Input: part model. Units: mm. Frame: model coordinates. A direction names the side the tool comes from. Round coordinates to 2 decimals unless told otherwise and drop trailing zeros. Loops run counter-clockwise (first coordinate to the right, second up) from the corner with the lowest first, then second, coordinate; pieces in that order, holes last. Notation, with made-up numbers: (-26, -22) -> (-9, -22) arc R10 ccw to (-9, -5) -> close; hole circle Ø1 at (-16.75, -0.75). An arc over 180 degrees is marked (long way). Answer as a JSON object with one key per item and string values.
```python
from build123d import *

# Parameters (mm, degrees)
SKETCH_1_R          = 2.1
SKETCH_1_R_2        = 5.02
SKETCH_1_R_3        = 2
SKETCH_1_R_4        = 9.52
EXTRUDE_1_DEPTH     = 4
SKETCH_3_W          = 46.2
SKETCH_3_H          = 3.817212264
EXTRUDE_2_DEPTH     = 4
SKETCH_2_R          = 2
SKETCH_2_R_2        = 1.5
SKETCH_2_W          = 32.809844138
SKETCH_2_H          = 42
SKETCH_2_W_2        = 8.2
SKETCH_2_H_2        = 4.2
CUT_EXTRUDE_1_DEPTH = 4
FILLET_1_R          = 2


with BuildPart() as part:
    # 草图1 → 凸台-拉伸1 (new body)
    with BuildSketch(Plane.XY):
        with BuildLine():
            ThreePointArc((-1.457142857, 39.854285714), (-41.457142857, -0.145714286), (-1.457142857, -40.145714286))
            Line((-1.457142857, -40.145714286), (328.542857143, -40.145714286))
            ThreePointArc((328.542857143, -40.145714286), (368.542857143, -0.145714286), (328.542857143, 39.854285714))
            Line((328.542857143, 39.854285714), (-1.457142857, 39.854285714))
        make_face()
        with Locations((-1.457142857, -23.895714286)):
            Circle(SKETCH_1_R, mode=Mode.SUBTRACT)
        with Locations((-20.942714442, -11.395714286)):
            Circle(SKETCH_1_R, mode=Mode.SUBTRACT)
        with Locations((18.028428728, -11.395714286)):
            Circle(SKETCH_1_R, mode=Mode.SUBTRACT)
        with Locations((-1.457142857, -0.145714286)):
            Circle(SKETCH_1_R_2, mode=Mode.SUBTRACT)
        with Locations((238.542857143, -16.645714286)):
            Circle(SKETCH_1_R_3, mode=Mode.SUBTRACT)
        with Locations((288.542857143, -0.145714286)):
            Circle(SKETCH_1_R_3, mode=Mode.SUBTRACT)
        with Locations((328.542857143, -0.145714286)):
            Circle(SKETCH_1_R_4, mode=Mode.SUBTRACT)
        with Locations((-22.025246197, 11.729285714)):
            Circle(SKETCH_1_R, mode=Mode.SUBTRACT)
        with Locations((19.110960483, 11.729285714)):
            Circle(SKETCH_1_R, mode=Mode.SUBTRACT)
        with Locations((-1.457142857, 22.354285714)):
            Circle(SKETCH_1_R, mode=Mode.SUBTRACT)
        with Locations((238.542857143, 16.354285714)):
            Circle(SKETCH_1_R_3, mode=Mode.SUBTRACT)
    extrude(amount=EXTRUDE_1_DEPTH)

    # 草图3 → 凸台-拉伸2 (add)
    with BuildSketch(Plane.XY.offset(4)):
        with Locations((18.542857143, -41.36131722)):
            Rectangle(SKETCH_3_W, SKETCH_3_H)
    extrude(amount=-EXTRUDE_2_DEPTH)

    # 草图2 → 切除-拉伸1 (cut)
    with BuildSketch(Plane.XY.offset(4)):
        with Locations((18.542857143, 33.854285714)):
            Circle(SKETCH_2_R)
        with Locations((108.542857143, 33.854285714)):
            Circle(SKETCH_2_R)
        with Locations((198.542857143, 33.854285714)):
            Circle(SKETCH_2_R)
        with Locations((288.542857143, 33.854285714)):
            Circle(SKETCH_2_R)
        with Locations((108.542857143, -34.145714286)):
            Circle(SKETCH_2_R)
        with Locations((198.542857143, -34.145714286)):
            Circle(SKETCH_2_R)
        with Locations((288.542857143, -34.145714286)):
            Circle(SKETCH_2_R)
        with Locations((18.542857143, -40.329923352)):
            Circle(SKETCH_2_R_2)
        Polygon((31.542857143, -21.145714286), (104.183898028, -21.145714286), (159.772133322, 20.854285714), (31.542857143, 20.854285714), align=None)
        Polygon((148.123425102, -21.145714286), (203.711660396, 20.854285714), (233.542857143, 20.854285714), (233.542857143, -21.145714286), align=None)
        with Locations((259.947779212, -0.145714286)):
            Rectangle(SKETCH_2_W, SKETCH_2_H)
        with Locations((33.542857143, -40.329923352)):
            Rectangle(SKETCH_2_W_2, SKETCH_2_H_2)
        with Locations((3.542857143, -40.329923352)):
            Rectangle(SKETCH_2_W_2, SKETCH_2_H_2)
    extrude(amount=-CUT_EXTRUDE_1_DEPTH, mode=Mode.SUBTRACT)

    # 圆角1
    fillet_1_edges = [part.edges().sort_by_distance(p)[0] for p in [
        (243.542857143, 20.854285714, 2),
        (276.352701281, 20.854285714, 2),
        (276.352701281, -21.145714286, 2),
        (243.542857143, -21.145714286, 2),
        (31.542857143, -21.145714286, 2),
        (31.542857143, 20.854285714, 2),
        (159.772133322, 20.854285714, 2),
        (104.183898028, -21.145714286, 2),
        (203.711660396, 20.854285714, 2),
        (233.542857143, 20.854285714, 2),
        (233.542857143, -21.145714286, 2),
        (148.123425102, -21.145714286, 2),
    ]]
    fillet(fillet_1_edges, radius=FILLET_1_R)


solid = part.part
```
1) Draft query along X for faces 1 (the face through (-41.385, 2.262, 1.972)), 2 (the face through (3.33, 1.36, 1.97)), 3 (the face through (368.533, -1.025, 1.972)). Return one class per face: +X half, -X half, draft (parallel to the pull), parting line (faces both ways), or undercut.
Output:
{"face 1": "-X half", "face 2": "undercut", "face 3": "+X half"}
2) Contact query for flat-ended pins moving along their axis: P1, Ø2.5, axis at x = 238.54, y = -16.65, coming from the +Z side; P2, Ø1, axis at y = 12, z = 3, coming from the +X side; P3, Ø1.2, axis at y = 5.5, z = 3, coming from the +X side; P4, Ø1.5, axis at y = 26, z = 0.5, coming from the +X side. Output: stop coordinate, or through.
Output:
{"P1": "passes through", "P2": "stops at x = 366.81", "P3": "stops at x = 368.22", "P4": "stops at x = 359.45"}
3) Section D-D, the plane z = 1.8. Count the separate pieces of the cut face and the enclosed holes in it, plus the area to 3 significant figures.
Output:
{"separate pieces": "1", "enclosed holes": "24", "area": "22,900 mm^2"}
4) Section C-C, the plane x = 170. Output: boundary loops of the cut face in (y, z), plus the area to 3 significant figures.
Output:
{"outline": "(-40.15, 0) -> (-21.15, 0) -> (-21.15, 4) -> (-40.15, 4) -> close; (-4.62, 0) -> (39.85, 0) -> (39.85, 4) -> (-4.62, 4) -> close", "area": "254 mm^2"}
5) Reachability of faces 4 (the face through (161, -1, 4)), 5 (the face through (129.51, -2.01, 2.03)) from +Z, -Z, +X, -X, +Y, -Y: full face, straight path, thin tool, end or side. Return the list, or none.
Output:
{"face 4": "+Z, +X, -X, +Y, -Y", "face 5": "+Z, -Z"}
6) Ray query, probe 1 along Y at (x, z) = (254.5, 2.3); probe 2 along Y at (x, z) = (-1, 2.2); probe 3 along X at (y, z) = (32.5, 3.3). Return the intervals inside material, ascending.
Output:
{"probe 1": "y = -40.15 to -21.15, 20.85 to 39.85", "probe 2": "y = -43.27 to -25.95, -21.85 to -5.14, 4.85 to 20.3, 24.4 to 39.85", "probe 3": "x = -24.57 to 17.07, 20.01 to 107.07, 110.01 to 197.07, 200.01 to 287.07, 290.01 to 351.66"}
7) Section B-B, the plane x = 313.5. Output: boundary loops of the cut face in (y, z), plus the area to 3 significant figures.
Output:
{"outline": "(-40.15, 0) -> (39.85, 0) -> (39.85, 4) -> (-40.15, 4) -> close", "area": "320 mm^2"}
8) Section A-A, the plane x = 256. Output: boundary loops of the cut face in (y, z).
Output:
{"outline": "(-40.15, 0) -> (-21.15, 0) -> (-21.15, 4) -> (-40.15, 4) -> close; (20.85, 0) -> (39.85, 0) -> (39.85, 4) -> (20.85, 4) -> close"}
